Model file for the job. Use its own axes, mm. Coordinates: 2 decimals unless noted, no trailing zeros. Loops run counter-clockwise (first coordinate to the right, second up) from the corner with the lowest first, then second, coordinate; pieces in that order, holes last.
from build123d import *

# Parameters (mm, degrees)
BLANKSKE_W         = 75
BLANKSKE_H         = 8.5
BLANK_DEPTH        = 10
TOOTHCUTSIM_DEPTH  = 77.139674284
TEETHCUTS_COUNT    = 25
TEETHCUTS_PITCH    = 3.14159265
SKETCH1_R          = 1.5
CUT_EXTRUDE1_DEPTH = 10


with BuildPart() as part:
    # BlankSke → Blank (new body)
    with BuildSketch(Plane.XY):
        with Locations((37.5, 4.25)):
            Rectangle(BLANKSKE_W, BLANKSKE_H)
    extrude(amount=-BLANK_DEPTH)

    # TooCutSkeSim → ToothCutSim (cut, through all)
    with BuildSketch(Plane.XY):
        Polygon((0.48943537, 6.25), (-0.48943537, 6.25), (-1.317613241, 8.5254), (1.317613241, 8.5254), align=None)
    toothcutsim = extrude(amount=-TOOTHCUTSIM_DEPTH, mode=Mode.SUBTRACT)

    # TeethCuts: ToothCutSim ×25
    with Locations(*[(i * TEETHCUTS_PITCH, 0, 0) for i in range(1, TEETHCUTS_COUNT)]):
        add(toothcutsim, mode=Mode.SUBTRACT)

    # Sketch1 → Cut-Extrude1 (cut)
    with BuildSketch(Plane.XY):
        with Locations((10, 3.125)):
            Circle(SKETCH1_R)
        with Locations((30, 3.125)):
            Circle(SKETCH1_R)
    extrude(amount=-CUT_EXTRUDE1_DEPTH, mode=Mode.SUBTRACT)


solid = part.part
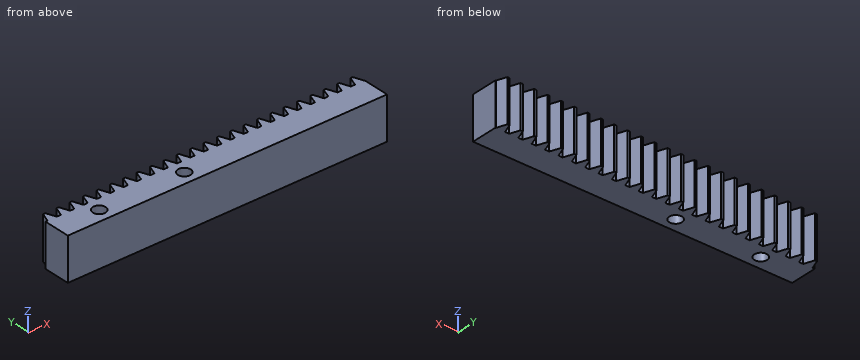
Q1. Slice it at B-B (z = -5.25). Count the separate pieces of the cut face and the enclosed holes in it, and give its area (3 significant figures).
Answers:
separate pieces: 1
enclosed holes: 2
area: 527 mm2
Q2. Flat gauge pin, fed straight in: P1, Ø0.8, axis at x = 66, z = -5.5, coming from the +Y side. Where does the tip first touch, or does it go through?
Answers:
P1: stops at y = 6.25
Q3. Drill centre lines: line 1 (X direction, y = 4.5, z = -6.75); line 2 (X direction, y = 2, z = -2.75); line 3 (Y direction, x = 30, z = -3.5) (3 decimals). Where is each one in solid material? Low to high.
Answers:
line 1: x = 0 to 9.4, 10.6 to 29.4, 30.6 to 75
line 2: x = 0 to 9.01, 10.99 to 29.01, 30.99 to 75
line 3: y = 0 to 1.625, 4.625 to 8.5
Q4. Slice it at A-A (y = 2.25). List the corners of the cut face in (x, z).
Answers:
outline: (0, -10) - (8.78, -10) - (8.78, 0) - (0, 0) - close; (11.22, -10) - (28.78, -10) - (28.78, 0) - (11.22, 0) - close; (31.22, -10) - (75, -10) - (75, 0) - (31.22, 0) - close
